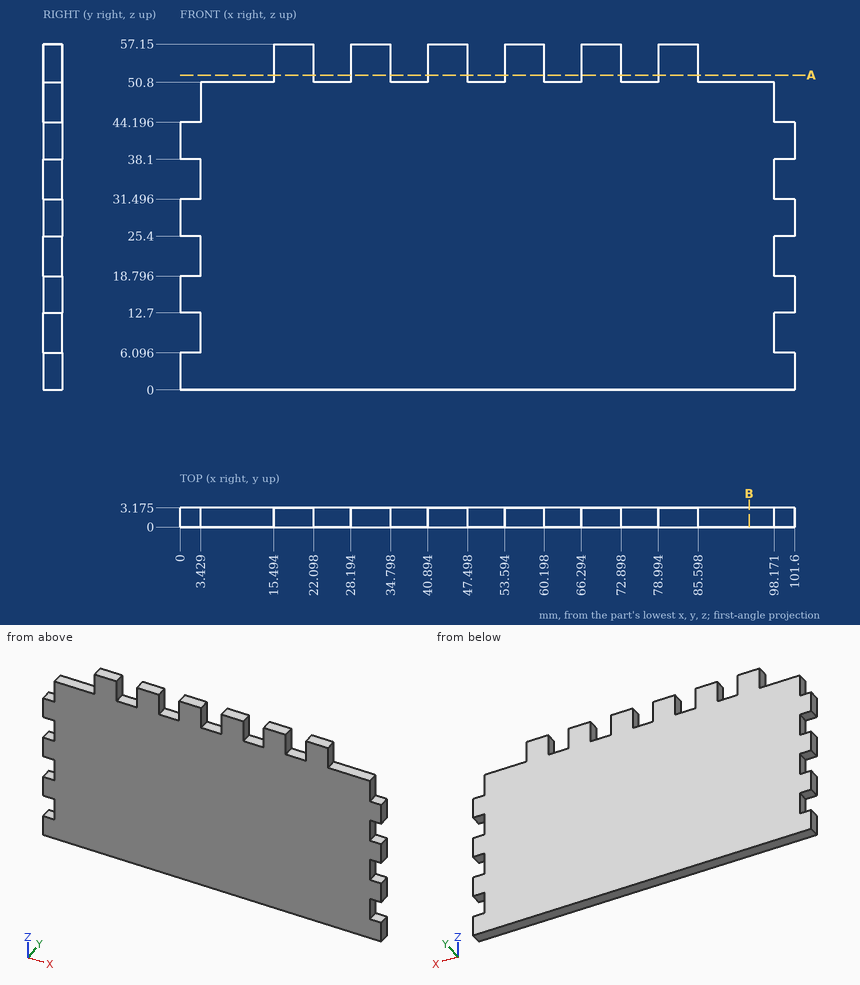
Could you check a few things on this drawing? It's one solid part, dimensions in mm from its lowest x, y, z. Round coordinates to 2 decimals unless told otherwise and drop trailing zeros. Write each loop counter-clockwise with the first axis right and the second up, starting at its lowest first coordinate (ties: lowest second). Pieces come first, ordered by that corner, then holes. Notation, with made-up numbers: (77.25, 24.25) -> (83.25, 24.25) arc R14 cw to (83.25, 39.25) -> close; hole circle Ø11 at (5, -8). An arc over 180 degrees is marked (long way). One line per item, written item: value.
1) Suppose I cut it at B-B on x = 94. List the corners of the cut face in (y, z) for me (3 decimals), plus the area to 3 significant figures.
Filled sheet:
outline: (0, 0) -> (3.175, 0) -> (3.175, 50.8) -> (0, 50.8) -> close
area: 161 mm2
2) Suppose I cut it at A-A on z = 52. List the corners of the cut face in (x, y) for me (3 decimals).
Filled sheet:
outline: (15.494, 0) -> (22.098, 0) -> (22.098, 3.175) -> (15.494, 3.175) -> close; (28.194, 0) -> (34.798, 0) -> (34.798, 3.175) -> (28.194, 3.175) -> close; (40.894, 0) -> (47.498, 0) -> (47.498, 3.175) -> (40.894, 3.175) -> close; (53.594, 0) -> (60.198, 0) -> (60.198, 3.175) -> (53.594, 3.175) -> close; (66.294, 0) -> (72.898, 0) -> (72.898, 3.175) -> (66.294, 3.175) -> close; (78.994, 0) -> (85.598, 0) -> (85.598, 3.175) -> (78.994, 3.175) -> close
3) If I drill on line 1 (X direction, y = 2.45, z = 54); line 2 (X direction, y = 2.3, z = 36); line 3 (Z direction, x = 15, y = 2.7), over which ranges is the centre line in solid material (lowest first)? Write a range as [from, to].
Filled sheet:
line 1: x = [15.49, 22.1], [28.19, 34.8], [40.89, 47.5], [53.59, 60.2], [66.29, 72.9], [78.99, 85.6]
line 2: x = [3.43, 98.17]
line 3: z = [0, 50.8]
4) I'm going to push flat-ended pins straight in: pin 1 Ø5 at (x, z) = (17, 19.5) entering from -Y; pin 2 Ø1 at (y, z) = (1.5, 54) entering from +X; pin 3 Ø1.6 at (x, y) = (94, 1.5) entering from +Z; pin 4 Ø1.6 at (x, y) = (100, 2) entering from +Z. Where does each tip first touch, or does it pass through?
Filled sheet:
pin 1: stops at y = 0
pin 2: stops at x = 85.6
pin 3: stops at z = 50.8
pin 4: stops at z = 44.2
